from build123d import *

# Parameters (mm, degrees)
BOSS_EXTRUDE1_DEPTH = 3.175
SKETCH3_R           = 2.38125
CUT_EXTRUDE1_DEPTH  = 5.08
SKETCH5_W           = 3.175
SKETCH5_H           = 12.7
BOSS_EXTRUDE2_DEPTH = 3.175


with BuildPart() as part:
    # Sketch1 → Boss-Extrude1 (new body)
    with BuildSketch(Plane.XY):
        Polygon((-38.1, 365.778475051), (-20.6375, 365.778475051), (-20.6375, 346.728475051), (-17.4625, 346.728475051), (-17.4625, 365.778475051), (0, 365.778475051), (0, 267.318840011), (-17.4625, 267.318840011), (-17.4625, 286.368840011), (-20.6375, 286.368840011), (-20.6375, 267.318840011), (-38.1, 267.318840011), align=None)
    extrude(amount=BOSS_EXTRUDE1_DEPTH)

    # Sketch3 → Cut-Extrude1 (cut)
    with BuildSketch(Plane.XY.offset(3.175)):
        with Locations((-19.05, 316.548657531)):
            Circle(SKETCH3_R)
        with BuildLine():
            ThreePointArc((-31.397852166, 304.200805365), (-19.05, 299.086157531), (-6.702147834, 304.200805365))
            ThreePointArc((-6.702147834, 304.200805365), (-6.702147834, 307.56840141), (-10.069743879, 307.56840141))
            ThreePointArc((-10.069743879, 307.56840141), (-19.05, 303.848657531), (-28.030256121, 307.56840141))
            ThreePointArc((-28.030256121, 307.56840141), (-31.397852166, 307.56840141), (-31.397852166, 304.200805365))
        make_face()
        with BuildLine():
            ThreePointArc((-6.702147834, 328.896509698), (-19.05, 334.011157531), (-31.397852166, 328.896509698))
            ThreePointArc((-31.397852166, 328.896509698), (-31.397852166, 325.528913652), (-28.030256121, 325.528913652))
            ThreePointArc((-28.030256121, 325.528913652), (-19.05, 329.248657531), (-10.069743879, 325.528913652))
            ThreePointArc((-10.069743879, 325.528913652), (-6.702147834, 325.528913652), (-6.702147834, 328.896509698))
        make_face()
    extrude(amount=-CUT_EXTRUDE1_DEPTH, mode=Mode.SUBTRACT)

    # Sketch5 → Boss-Extrude2 (add)
    with BuildSketch(Plane.XY.offset(3.175)):
        with Locations((1.5875, 336.36769286)):
            Rectangle(SKETCH5_W, SKETCH5_H)
        with Locations((1.5875, 304.329924583)):
            Rectangle(SKETCH5_W, SKETCH5_H)
        with Locations((-39.6875, 304.329924583)):
            Rectangle(SKETCH5_W, SKETCH5_H)
        with Locations((-39.6875, 336.36769286)):
            Rectangle(SKETCH5_W, SKETCH5_H)
    extrude(amount=-BOSS_EXTRUDE2_DEPTH)


solid = part.part
Could you check a few things on this model? Use its own coordinates, in mm. A direction names the side the tool comes from. Round coordinates to 2 decimals unless told otherwise and drop trailing zeros. Write each loop counter-clockwise with the first axis right and the second up, starting at its lowest first coordinate (ties: lowest second). Pieces come first, ordered by that corner, then holes. Notation, with made-up numbers: (-13.75, 73.5) -> (40.25, 73.5) arc R19 ccw to (40.25, 110.5) -> close; hole circle Ø7 at (89.25, 11). An arc over 180 degrees is marked (long way). Use a Markdown table: item, result.
1. If we section it at A-A (y = 276): List the corners of the cut face in (x, z) for me (1 decimal), then the cut area to 3 significant figures.
Answer key:
| item | result |
|---|---|
| outline | (-38.1, 0) -> (-20.6, 0) -> (-20.6, 3.2) -> (-38.1, 3.2) -> close; (-17.5, 0) -> (0, 0) -> (0, 3.2) -> (-17.5, 3.2) -> close |
| area | 111 mm^2 |
2. If we section it at C-C (x = -30.5): List the corners of the cut face in (y, z) for me (3 decimals), then the cut area to 3 significant figures.
Answer key:
| item | result |
|---|---|
| outline | (267.319, 0) -> (303.364, 0) -> (303.364, 3.175) -> (267.319, 3.175) -> close; (308.132, 0) -> (324.965, 0) -> (324.965, 3.175) -> (308.132, 3.175) -> close; (329.733, 0) -> (365.778, 0) -> (365.778, 3.175) -> (329.733, 3.175) -> close |
| area | 282 mm^2 |
3. If we section it at D-D (y = 289): List the corners of the cut face in (x, z) for me (3 decimals).
Answer key:
| item | result |
|---|---|
| outline | (-38.1, 0) -> (0, 0) -> (0, 3.175) -> (-38.1, 3.175) -> close |
4. If we section it at B-B (x = -19.05): List the corners of the cut face in (y, z) for me (3 decimals).
Answer key:
| item | result |
|---|---|
| outline | (286.369, 0) -> (299.086, 0) -> (299.086, 3.175) -> (286.369, 3.175) -> close; (303.849, 0) -> (314.167, 0) -> (314.167, 3.175) -> (303.849, 3.175) -> close; (318.93, 0) -> (329.249, 0) -> (329.249, 3.175) -> (318.93, 3.175) -> close; (334.011, 0) -> (346.728, 0) -> (346.728, 3.175) -> (334.011, 3.175) -> close |
5. Please list where these lines run through material, in increasing order: probe 1 along Y at (x, z) = (-19.05, 1.45); probe 2 along Y at (x, z) = (-15.5, 2.8); probe 3 along X at (y, z) = (281, 0.5).
Answer key:
| item | result |
|---|---|
| probe 1 | y = 286.37 to 299.09, 303.85 to 314.17, 318.93 to 329.25, 334.01 to 346.73 |
| probe 2 | y = 267.32 to 299.45, 304.35 to 328.74, 333.65 to 365.78 |
| probe 3 | x = -38.1 to -20.64, -17.46 to 0 |
6. Which directions (+Z, -Z, +X, -X, +Y, -Y) give clear straight access to the entire face, cutting with the end or side of a thin tool? Please do faces 4 (the face through (-18.86, 334.01, 1.61)), 5 (the face through (-17.462, 277, 2)), 6 (the face through (-19, 346.728, 2)), 7 (the face through (2, 342.718, 2)).
Answer key:
| item | result |
|---|---|
| face 4 | +Z, -Z |
| face 5 | +Z, -Z, -Y |
| face 6 | +Z, -Z, +Y |
| face 7 | +Z, -Z, +X, +Y |
7. For pin 1 Ø1.6 at (x, z) = (-39.5, 1) entering from +Y; pin 2 Ø1.6 at (y, z) = (358.5, 2) entering from +X; pin 3 Ø1 at (y, z) = (353, 1) entering from -X, each with a flat end and sliding along its axis, tell me the tip position at first contact or that it passes through.
Answer key:
| item | result |
|---|---|
| pin 1 | stops at y = 342.72 |
| pin 2 | stops at x = 0 |
| pin 3 | stops at x = -38.1 |
8. We'd pull the mould along X, two halves only. Please class faces 1 (the face through (-29, 365.778, 2)), 2 (the face through (-19, 286.369, 2)), 3 (the face through (0, 283, 2)): +X half, -X half, draft (parallel to the pull), parting line (faces both ways), or undercut.
Answer key:
| item | result |
|---|---|
| face 1 | draft |
| face 2 | undercut |
| face 3 | +X half |
